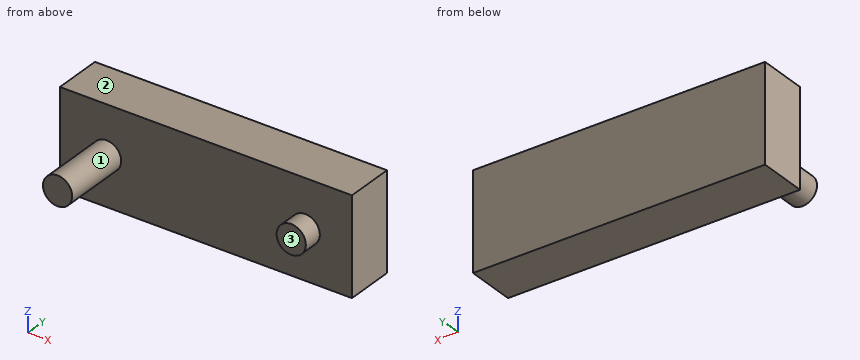
from build123d import *

# Parameters (mm, degrees)
F0_W     = 38.1
F0_H     = 12.7
F1_DEPTH = 6.35
F2_R     = 1.905
F3_DEPTH = 8.89
F4_R     = 1.905
F5_DEPTH = 2.54


with BuildPart() as f1:
    # F0 (on Front) → F1 (new body)
    with BuildSketch(Plane.XZ):
        Rectangle(F0_W, F0_H)
    extrude(amount=F1_DEPTH)

    # F2 (on face) → F3 (join)
    with BuildSketch(Plane.XZ.offset(6.35)):
        with Locations((-12.954, 0)):
            Circle(F2_R)
    extrude(amount=F3_DEPTH)

    # F4 (on face) → F5 (join)
    with BuildSketch(Plane.XZ.offset(6.35)):
        with Locations((12.954, 0)):
            Circle(F4_R)
    extrude(amount=F5_DEPTH)


solid = f1.part
Verification items for the finished model (mm, model axes). Face numbers are marked on the shaded views. A direction names the side the tool comes from. Coordinates: 2 decimals unless noted, no trailing zeros. Order: outer loops, then holes, each group sorted by start corner. A loop starts at its lowest first (then second) coordinate and runs counter-clockwise, first axis right, second up.
1. Set-up check for the marked faces 1, 2 and 3: record each of +Z, -Z, +X, -X, +Y, -Y from which the full face is reachable in a straight line by a thin tool's end or side.
Results found:
face 1: -Y
face 2: +Z, +X, -X, +Y, -Y
face 3: +Z, -Z, +X, -Y
2. Sectioned sample at C-C, the plane y = -11.25. Record the cut outline in (x, z) (3 decimals), and give its area (3 significant figures).
Results found:
outline: circle Ø3.81 at (-12.954, 0)
area: 11.4 mm2
3. Scan lines: line 1 (Y direction, x = 16.5, z = 2.5); line 2 (Z direction, x = -13, y = -8.25); line 3 (Y direction, x = 12, z = 1). Record each from-to range of solid material in increasing order.
Results found:
line 1: y = -6.35 to 0
line 2: z = -1.9 to 1.9
line 3: y = -8.89 to 0
4. Sectioned sample at D-D, the plane x = -0.5. Record the cut outline in (y, z), and give its area (3 significant figures).
Results found:
outline: (-6.35, -6.35) - (0, -6.35) - (0, 6.35) - (-6.35, 6.35) - close
area: 80.6 mm2
5. Sectioned sample at A-A, the plane z = 0. Record the cut outline in (x, y).
Results found:
outline: (-19.05, -6.35) - (-14.86, -6.35) - (-14.86, -15.24) - (-11.05, -15.24) - (-11.05, -6.35) - (11.05, -6.35) - (11.05, -8.89) - (14.86, -8.89) - (14.86, -6.35) - (19.05, -6.35) - (19.05, 0) - (-19.05, 0) - close
6. Sectioned sample at B-B, the plane y = -7.5. Record the cut outline in (x, z) (3 decimals).
Results found:
outline: circle Ø3.81 at (-12.954, 0); circle Ø3.81 at (12.954, 0)
7. Go/stop test with flat-tipped pins: pin 1 Ø3 at (x, z) = (12.5, -0.5) entering from -Y; pin 2 Ø1 at (x, z) = (-2.5, 4.5) entering from -Y; pin 3 Ø5 at (x, y) = (-13.5, -10) entering from +Z (3 decimals). Record where each tip stops, or that it passes through.
Results found:
pin 1: stops at y = -8.89
pin 2: stops at y = -6.35
pin 3: stops at z = 1.905
